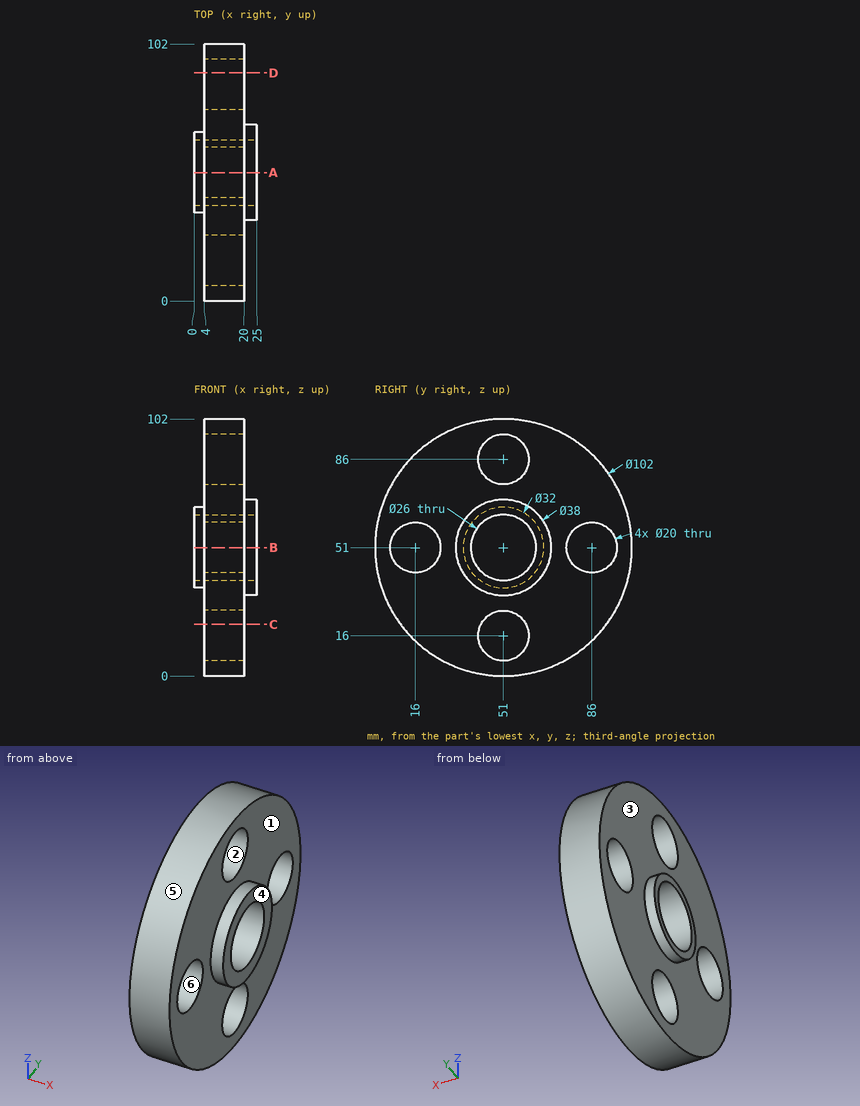
The figure shows three views and two pictorial views of one solid part (mm, origin at its lowest corner). Answer the questions. A direction names the side the tool comes from. Round coordinates to 2 decimals unless told otherwise and drop trailing zeros. Loops run counter-clockwise (first coordinate to the right, second up) from the corner with the lowest first, then second, coordinate; pieces in that order, holes last. Notation, with made-up numbers: (45.5, 11) - (66.5, 11) arc R20 ccw to (66.5, 25) - close; hole circle Ø7 at (-20, 63). An arc over 180 degrees is marked (long way). Use one line per item in the form item = value. Start each with the question number.
(1) Find section A-A on y = 51. Determine the outline of the cut face in (x, z), and give its area (3 significant figures).
(2) Find section D-D on y = 90.5. Determine the outline of the cut face in (x, z).
(3) Determine the mould class of the marked faces 4, 5 and 6 for opening direction Y: +Y half, -Y half, draft (parallel to the pull), parting line (faces both ways), or undercut.
(4) Flat-ended cylindrical pins translate along their axes: P1, Ø1, axis at x = 9, y = 13.5, coming from the -Z side; P2, Ø2, axis at x = 15, z = 66.5, coming from the +Y side; P3, Ø23, axis at y = 51, z = 16, coming from the -X side; P4, Ø21, axis at y = 51, z = 51, coming from the +X side. Find the tip coordinate at first contact, or state that the pin passes through.
(5) Which of the six approach directions +Z, -Z, +X, -X, +Y, -Y give full straight-line access (tool end or side, diameter ignored) to the marked faces 1, 2 and 3?
(6) Find section C-C on z = 20.5. Determine the outline of the cut face in (x, y).
(7) Consider line 1 (Z direction, x = 12.25, y = 51); line 2 (Y direction, x = 3, z = 51); line 3 (Y direction, x = 4.25, z = 52.5). Determine where each line is inside the solid, lowest interval first.
Answer list:
q1.outline = (0, 35) - (4, 35) - (4, 26) - (20, 26) - (20, 32) - (25, 32) - (25, 38) - (0, 38) - close; (0, 64) - (25, 64) - (25, 70) - (20, 70) - (20, 76) - (4, 76) - (4, 67) - (0, 67) - close; (4, 0) - (20, 0) - (20, 6) - (4, 6) - close; (4, 96) - (20, 96) - (20, 102) - (4, 102) - close
q1.area = 660 mm^2
q2.outline = (4, 18.74) - (20, 18.74) - (20, 42.07) - (4, 42.07) - close; (4, 59.93) - (20, 59.93) - (20, 83.26) - (4, 83.26) - close
q3.face_4 = draft
q3.face_5 = parting line
q3.face_6 = undercut
q4.P1 = 15.9
q4.P2 = 99.9
q4.P3 = 4
q4.P4 = through
q5.face_1 = +X
q5.face_2 = +X, -X
q5.face_3 = -X
q6.outline = (4, 10.13) - (20, 10.13) - (20, 42.07) - (4, 42.07) - close; (4, 59.93) - (20, 59.93) - (20, 91.87) - (4, 91.87) - close
q7.line_1 = 0 to 6, 26 to 38, 64 to 76, 96 to 102
q7.line_2 = 35 to 38, 64 to 67
q7.line_3 = 0.02 to 6.11, 25.89 to 38.09, 63.91 to 76.11, 95.89 to 101.98
